Geometry: final body of the model. Coordinates: model frame, mm. A direction names the side the tool comes from. Round coordinates to 2 decimals unless told otherwise and drop trailing zeros. Loops run counter-clockwise (first coordinate to the right, second up) from the corner with the lowest first, then second, coordinate; pieces in that order, holes last. Notation, with made-up numbers: (61.25, 86) - (114.25, 86) arc R29 ccw to (114.25, 109) - close; hole circle Ø3 at (65, -14). An arc over 180 degrees is marked (long way). Return JSON: item names as keys, results as strings. Group by question number.
1. Section B-B on y = -2.5. Count the separate pieces of the cut face and the enclosed holes in it, and give its area (3 significant figures).
2. Section A-A on z = 8.25. Return loops of the section in (x, y), and give its area (3 significant figures).
3. Set-up query: faces 1 (the face through (13, -1, 0)), 2 (the face through (-1.93, -8.68, 10.12)). Return all of +Z, -Z, +X, -X, +Y, -Y with unobstructed straight access to the full face (end or side cutting, diameter ignored); none if empty.
4. First-contact query: pin 1 Ø14 at (x, y) = (-2.5, -3.5) entering from +Z; pin 2 Ø6 at (x, z) = (7.5, 11) entering from -Y; pin 3 Ø1 at (y, z) = (-11.5, 11) entering from +X; pin 4 Ø8 at (x, y) = (30.48, 0) entering from -Z. Flat tips, straight axial feed; report the tip coordinate or a pass-through.
5. Material intervals for probe 1 along Y at (x, z) = (0, 10.2); probe 2 along X at (y, z) = (3.5, 13); probe 3 along Y at (x, z) = (30.48, 9.4), sorted ascending.
6. Draft query along X for faces 3 (the face through (-1.173, 8.937, 12.823)), 4 (the face through (38, 3, 15.24)), 5 (the face through (18.05, -11.93, 3.86)). Return one class per face: +X half, -X half, draft (parallel to the pull), parting line (faces both ways), or undercut.
from build123d import *

# Parameters (mm, degrees)
F0_R     = 8.89
F0_R_2   = 5.08
F1_DEPTH = 7.62
F1_TAPER = -3
F2_R     = 15.24
F2_R_2   = 8.89
F2_R_3   = 5.08
F3_DEPTH = 7.62
F4_SIZE  = 2.54


with BuildPart() as f1:
    # F0 (on Top) → F1 (new body)
    with BuildSketch(Plane.XY):
        with BuildLine():
            ThreePointArc((4.0809852702, -14.6834314526), (12.1336683554, -9.2212630502), (15.24, 0))
            ThreePointArc((15.24, 0), (11.8457713974, 9.5882897328), (3.175, 14.9056021348))
            ThreePointArc((3.175, 14.9056021348), (-15.2323925132, 0.4814751535), (2.2273110086, -15.0763618181))
            Line((2.2273110086, -15.0763618181), (4.0809852702, -14.6834314526))
        make_face()
        Circle(F0_R, mode=Mode.SUBTRACT)
        with BuildLine():
            ThreePointArc((39.37, 0), (37.3900333152, 5.5931690108), (32.3320833333, 8.6949345786))
            ThreePointArc((32.3320833333, 8.6949345786), (21.5900010863, 0.0043948805), (32.323485534, -8.6967615286))
            ThreePointArc((32.323485534, -8.6967615286), (37.3872674191, -5.5965843871), (39.37, 0))
        make_face()
        with Locations((30.48, 0)):
            Circle(F0_R_2, mode=Mode.SUBTRACT)
        with BuildLine():
            ThreePointArc((3.175, 14.9056021348), (11.8457713974, 9.5882897328), (15.24, 0))
            ThreePointArc((15.24, 0), (12.1336683554, -9.2212630502), (4.0809852702, -14.6834314526))
            Line((4.0809852702, -14.6834314526), (32.323485534, -8.6967615286))
            ThreePointArc((32.323485534, -8.6967615286), (21.5900010863, 0.0043948805), (32.3320833333, 8.6949345786))
            Line((32.3320833333, 8.6949345786), (3.175, 14.9056021348))
        make_face()
    extrude(amount=F1_DEPTH, taper=F1_TAPER)

    # F2 (on face) → F3 (join)
    with BuildSketch(Plane.XY.offset(7.62)):
        Circle(F2_R)
        Circle(F2_R_2, mode=Mode.SUBTRACT)
        with Locations((30.48, 0)):
            Circle(F2_R_2)
        with Locations((30.48, 0)):
            Circle(F2_R_3, mode=Mode.SUBTRACT)
    extrude(amount=F3_DEPTH)

    # F4
    f4_edges = [f1.edges().sort_by_distance(p)[0] for p in [
        (-8.89, 0, 15.24),
        (25.4, 0, 15.24),
    ]]
    chamfer(f4_edges, length=F4_SIZE)


solid = f1.part
Taken from the geometry:
{
 "1": {"separate pieces": "3", "enclosed holes": "0", "area": "372 mm2"},
 "2": {"outline": "circle Ø30.48 at (0, 0); circle Ø17.78 at (30.48, 0); hole circle Ø17.78 at (0, 0); hole circle Ø10.16 at (30.48, 0)", "area": "649 mm2"},
 "3": {"face 1": "-Z, +X, -X, +Y, -Y", "face 2": "+Z"},
 "4": {"pin 1": "z = 15.11", "pin 2": "y = -14.56", "pin 3": "x = 10.55", "pin 4": "through"},
 "5": {"probe 1": "-15.24 to -8.89, 8.89 to 15.24", "probe 2": "-14.83 to -8.5, 8.5 to 14.83, 22.31 to 26.39, 34.57 to 38.65", "probe 3": "-8.89 to -5.08, 5.08 to 8.89"},
 "6": {"face 3": "undercut", "face 4": "draft", "face 5": "+X half"}
}
